Check sheet for the modelled part. Datum: model origin and axes. Units: mm. Face numbers are marked on the shaded views. A direction names the side the tool comes from. Round coordinates to 2 decimals unless told otherwise and drop trailing zeros. Order: outer loops, then holes, each group sorted by start corner. A loop starts at its lowest first (then second) coordinate and runs counter-clockwise, first axis right, second up. Notation, with made-up numbers: M 58.5,-27 L 79.5,-27 A21 ccw 79.5,3 Z; hole C 67,76.25 d2. An arc over 180 degrees is marked long. One line per item, written item: value. Start each with the question number.
(1) Cross-section at C-C, the plane y = 17. Enter the section's corners in (x, z), and give its area (3 significant figures).
(2) Access from +Z, -Z, +X, -X, +Y, -Y to the whole of each face (thin tool, end or side, straight path). Record for the marked faces 1 and 2.
(3) Cross-section at D-D, the plane x = -23. Enter the section's corners in (y, z), and give its area (3 significant figures).
(4) Release check for a two-part mould opening along Z. For the marked faces 3, 4, 5 and 6 record: released by +Z, released by -Z, zero draft, split by the parting line, or undercut.
(5) Cross-section at B-B, the plane x = -31.5. Enter the section's corners in (y, z).
(6) Depth check by flat-ended pin: pin 1 Ø2 at (x, z) = (-18, 11.5) entering from +Y; pin 2 Ø4 at (x, y) = (-21.5, 2) entering from +Z; pin 3 Ø10 at (y, z) = (33, 27) entering from -X; pin 4 Ø3 at (x, z) = (-26, 18) entering from -Y. Enter the tip coordinate at first touch or a pass-through.
(7) Thickness scan on L1, parallel to Z at x = -36, y = -16; L2, parallel to X at y = 45.5, z = 18.5; L3, parallel to X at y = 24.5, z = 22.5. Record the ranges inside material, lowest first.
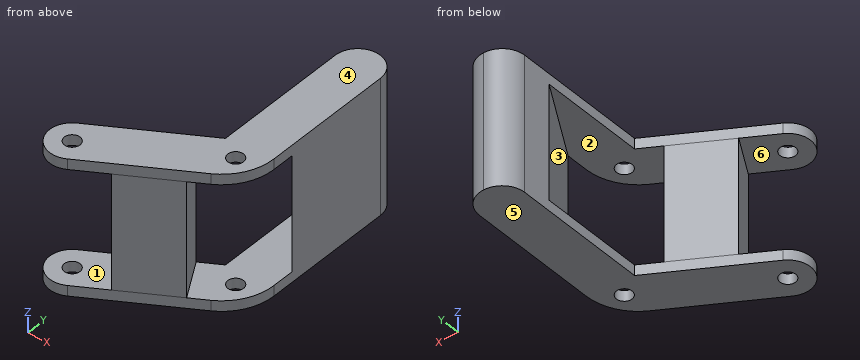
from build123d import *

# Parameters (mm, degrees)
SKETCH1_R           = 2.25
BOSS_EXTRUDE1_DEPTH = 39
SKETCH2_W           = 55
SKETCH2_H           = 33
CUT_EXTRUDE1_DEPTH  = 81.036070374
FILLET1_R           = 6.5
FILLET2_R           = 15
BOSS_EXTRUDE2_REACH = 76.379
FILLET3_R           = 6.5


with BuildPart() as part:
    # Sketch1 → Boss-Extrude1 (new body)
    with BuildSketch(Plane.XY):
        Polygon((7.10189894, 0.127356388), (7.308909237, 52.632501802), (-5.690989724, 52.683756073), (-5.868408354, 7.684105823), (-40.588007992, -12.179161807), (-34.132446013, -23.46303169), align=None)
        with Locations((-31.718292061, -14.593315758)):
            Circle(SKETCH1_R, mode=Mode.SUBTRACT)
        with Locations((0.306965546, 3.728504465)):
            Circle(SKETCH1_R, mode=Mode.SUBTRACT)
    extrude(amount=BOSS_EXTRUDE1_DEPTH)

    # Sketch2 → Cut-Extrude1 (cut, through all)
    with BuildSketch(Plane(origin=(1.696387072, -2.965165705, 0), x_dir=(0.8679899909572786, 0.49658169075992264, 0), z_dir=(0.4965816907599227, -0.8679899909572787, 0))):
        with Locations((-13.777933453, 19.5)):
            Rectangle(SKETCH2_W, SKETCH2_H)
    extrude(amount=-CUT_EXTRUDE1_DEPTH, mode=Mode.SUBTRACT)

    # Fillet1
    fillet1_edges = [part.edges().sort_by_distance(p)[0] for p in [
        (-34.132446013, -23.46303169, 1.5),
        (-40.588007992, -12.179161807, 1.5),
        (-34.132446013, -23.46303169, 37.5),
        (-40.588007992, -12.179161807, 37.5),
    ]]
    fillet(fillet1_edges, radius=FILLET1_R - 0.0001)  # a hair under: the kernel refuses the full size

    # Fillet2
    fillet2_edges = [part.edges().sort_by_distance(p)[0] for p in [
        (7.10189894, 0.127356388, 37.5),
        (7.10189894, 0.127356388, 1.5),
    ]]
    fillet(fillet2_edges, radius=FILLET2_R)

    # Sketch3 → Boss-Extrude2 (add, up to next)
    with BuildSketch(Plane.XY.offset(3), mode=Mode.PRIVATE) as boss_extrude2_sk1:
        Polygon((-26.266173142, -3.98556391), (-19.810611162, -15.269433792), (-5.145153373, -6.879247384), (-11.600715353, 4.404622498), align=None)
    boss_extrude2_tool1 = extrude(boss_extrude2_sk1.sketch, amount=BOSS_EXTRUDE2_REACH, mode=Mode.PRIVATE) - part.part
    add(boss_extrude2_tool1.solids().sort_by_distance((-15.705663, -5.432406, 3))[0])

    # Fillet3
    fillet3_edges = [part.edges().sort_by_distance(p)[0] for p in [
        (7.308909237, 52.632501802, 19.5),
        (-5.690989724, 52.683756073, 19.5),
    ]]
    fillet(fillet3_edges, radius=FILLET3_R - 0.0001)  # a hair under: the kernel refuses the full size


solid = part.part
Values found:
1. outline: M -5.83,0 L 7.17,0 L 7.17,39 L -5.83,39 L -5.83,36 L 6.08,36 L 6.08,3 L -5.83,3 Z
1. area: 114 mm^2
2. face 1: -X, -Y
2. face 2: none
3. outline: M -17.09,0 L -2.12,0 L -2.12,39 L -17.09,39 L -17.09,36 L -9.69,36 L -9.69,3 L -17.09,3 Z
3. area: 340 mm^2
4. face 3: undercut
4. face 4: released by +Z
4. face 5: released by -Z
4. face 6: undercut
5. outline: M -21.09,0 L -16.83,0 L -16.83,3 L -21.09,3 Z; M -21.09,36 L -16.83,36 L -16.83,39 L -21.09,39 Z; M -12.35,0 L -6.98,0 L -6.98,3 L -12.35,3 Z; M -12.35,36 L -6.98,36 L -6.98,39 L -12.35,39 Z
6. pin 1: y = 1.32
6. pin 2: through
6. pin 3: x = -5.75
6. pin 4: y = -7.07
7. L1: 0 to 3, 36 to 39
7. L2: -5.72 to 7.28
7. L3: 1.79 to 7.2
